from build123d import *

# Parameters (mm, degrees)
BOSS_EXTRUDE1_DEPTH = 25.4
CUT_EXTRUDE1_REACH  = 84.87
SKETCH2_R           = 0.99949
SKETCH2_W           = 22.86
SKETCH2_H           = 15.24
SKETCH3_W           = 12.7
SKETCH3_H           = 45.72
SKETCH3_R           = 2
BOSS_EXTRUDE2_DEPTH = 2.54


with BuildPart() as part:
    # Sketch1 → Boss-Extrude1 (new body)
    with BuildSketch(Plane.XY):
        with BuildLine():
            Line((-32.578270726, 40.408843429), (-59.736149583, 54.246473861))
            Line((-59.736149583, 54.246473861), (-58.583013714, 56.509630432))
            Line((-58.583013714, 56.509630432), (-31.425134857, 42.672))
            ThreePointArc((-31.425134857, 42.672), (-9.813641153, 25.020432537), (2.54, 0))
            Line((2.54, 0), (0, 0))
            ThreePointArc((0, 0), (-11.97175713, 23.685162685), (-32.578270726, 40.408843429))
        make_face()
    extrude(amount=BOSS_EXTRUDE1_DEPTH)

    # Sketch2 → Cut-Extrude1 (cut, up to next)
    with BuildSketch(Plane(origin=(10.784234574, 21.165252068, 0), x_dir=(0.8910065241883675, -0.45399049973954775, 0), z_dir=(0.45399049973954775, 0.8910065241883675, 0)), mode=Mode.PRIVATE) as cut_extrude1_sk1:
        with Locations(Location((-71.502682786, -2.41681, 0), (0, 0, 180))):
            Circle(SKETCH2_R)
    cut_extrude1_tool1 = extrude(cut_extrude1_sk1.sketch, amount=-CUT_EXTRUDE1_REACH, mode=Mode.PRIVATE) & part.part
    # Sketch2 → Cut-Extrude1 (cut, up to next)
    with BuildSketch(Plane(origin=(10.784234574, 21.165252068, 0), x_dir=(0.8910065241883675, -0.45399049973954775, 0), z_dir=(0.45399049973954775, 0.8910065241883675, 0)), mode=Mode.PRIVATE) as cut_extrude1_sk2:
        with Locations(Location((-71.502682786, -23.03399, 0), (0, 0, 180))):
            Circle(SKETCH2_R)
    cut_extrude1_tool2 = extrude(cut_extrude1_sk2.sketch, amount=-CUT_EXTRUDE1_REACH, mode=Mode.PRIVATE) & part.part
    # Sketch2 → Cut-Extrude1 (cut, up to next)
    with BuildSketch(Plane(origin=(10.784234574, 21.165252068, 0), x_dir=(0.8910065241883675, -0.45399049973954775, 0), z_dir=(0.45399049973954775, 0.8910065241883675, 0)), mode=Mode.PRIVATE) as cut_extrude1_sk3:
        with Locations((-62.307882786, -12.7)):
            Rectangle(SKETCH2_W, SKETCH2_H)
    cut_extrude1_tool3 = extrude(cut_extrude1_sk3.sketch, amount=-CUT_EXTRUDE1_REACH, mode=Mode.PRIVATE) & part.part
    add(cut_extrude1_tool1.solids().sort_by_distance((-52.925122, 53.626791, 2.41681))[0], mode=Mode.SUBTRACT)
    add(cut_extrude1_tool2.solids().sort_by_distance((-52.925122, 53.626791, 23.03399))[0], mode=Mode.SUBTRACT)
    add(cut_extrude1_tool3.solids().sort_by_distance((-44.732495, 49.452439, 12.7))[0], mode=Mode.SUBTRACT)

    # Sketch3 → Boss-Extrude2 (add)
    with BuildSketch(Plane(origin=(0, 0, 0), x_dir=(1, 0, 0), z_dir=(0, 1, 0))):
        with Locations((-3.81, -12.7)):
            Rectangle(SKETCH3_W, SKETCH3_H)
        with Locations(Location((-3.81, 6.35, 0), (0, 0, 270))):
            Circle(SKETCH3_R, mode=Mode.SUBTRACT)
        with Locations(Location((-3.81, -31.75, 0), (0, 0, 270))):
            Circle(SKETCH3_R, mode=Mode.SUBTRACT)
    extrude(amount=BOSS_EXTRUDE2_DEPTH)


solid = part.part
Check sheet for the modelled part. Datum: model origin and axes. Units: mm. A direction names the side the tool comes from. Round coordinates to 2 decimals unless told otherwise and drop trailing zeros. Loops run counter-clockwise (first coordinate to the right, second up) from the corner with the lowest first, then second, coordinate; pieces in that order, holes last.
1. Sectioned sample at A-A on z = -6.35. Record the boundary of the cut face in (x, y).
2. Sectioned sample at C-C on x = -38.5. Record the boundary of the cut face in (y, z), and give its area (3 significant figures).
3. Gauge pin test, flat ends, axial feed: pin 1 Ø1.5 at (y, z) = (22, 4.5) entering from -X; pin 2 Ø2 at (y, z) = (1.5, 14.5) entering from -X; pin 3 Ø4 at (x, y) = (-44.5, 49) entering from +Z; pin 4 Ø5 at (y, z) = (34, -4) entering from -X. Record the tip position at first contact, or that the pin passes through.
4. Sectioned sample at D-D on x = -11. Record the boundary of the cut face in (y, z), and give its area (3 significant figures).
5. Set-up check for faces 1 (the flat face through (-4, 0, 12)), 2 (the flat face through (-55.5, 53.5, 12.8)), 3 (the flat face through (-10.16, 1, 13)), 4 (the flat face through (-24, 36, 0)): record each of +Z, -Z, +X, -X, +Y, -Y from which the full face is reachable in a straight line by a thin tool's end or side.
6. Sectioned sample at B-B on x = -3.81. Record the boundary of the cut face in (y, z).
7. Mould release check, pull along X, two halves, no side actions. Record for faces 5 (the flat face through (-24, 36, 25.4)), 6 (the cylindrical face through (-12.58, 24.43, 12.52)), 7 (the cylindrical face through (-53.3, 52.41, 22.06)), 8 (the cylindrical face through (-3.722, 1.252, -8.348)): released by +X, released by -X, zero draft, split by the parting line, or undercut.
8. Scan lines: probe 1 along Z at (x, y) = (-3, 1); probe 2 along X at (y, z) = (1.6, 31.75); probe 3 along Y at (x, z) = (-7, -7.5). Record each from-to range of solid material in increasing order.
Recorded:
1. outline: (-10.16, 0) - (-5.81, 0) - (-5.81, 2.54) - (-10.16, 2.54) - close; (-1.81, 0) - (2.54, 0) - (2.54, 2.54) - (-1.81, 2.54) - close
2. outline: (43.43, 0) - (46.28, 0) - (46.28, 5.08) - (43.43, 5.08) - close; (43.43, 20.32) - (46.28, 20.32) - (46.28, 25.4) - (43.43, 25.4) - close
2. area: 29.0 mm2
3. pin 1: stops at x = -11.23
3. pin 2: stops at x = -10.16
3. pin 3: stops at z = 25.4
3. pin 4: passes through
4. outline: (22.45, 0) - (26.47, 0) - (26.47, 25.4) - (22.45, 25.4) - close
4. area: 102 mm2
5. face 1: +Z, -Z, +X, -X, -Y
5. face 2: +X, -Y
5. face 3: +Z, -Z, -X, -Y
5. face 4: -Z, +X, -X, +Y
6. outline: (0, -10.16) - (2.54, -10.16) - (2.54, -8.35) - (0, -8.35) - close; (0, -4.35) - (2.54, -4.35) - (2.54, 29.75) - (0, 29.75) - close; (0, 33.75) - (2.54, 33.75) - (2.54, 35.56) - (0, 35.56) - close; (10.57, 0) - (16.06, 0) - (16.06, 25.4) - (10.57, 25.4) - close
7. face 5: zero draft
7. face 6: released by -X
7. face 7: undercut
7. face 8: undercut
8. probe 1: z = -10.16 to -8.18, -4.52 to 29.92, 33.58 to 35.56
8. probe 2: x = -10.16 to -5.81, -1.81 to 2.54
8. probe 3: y = 0 to 2.54
